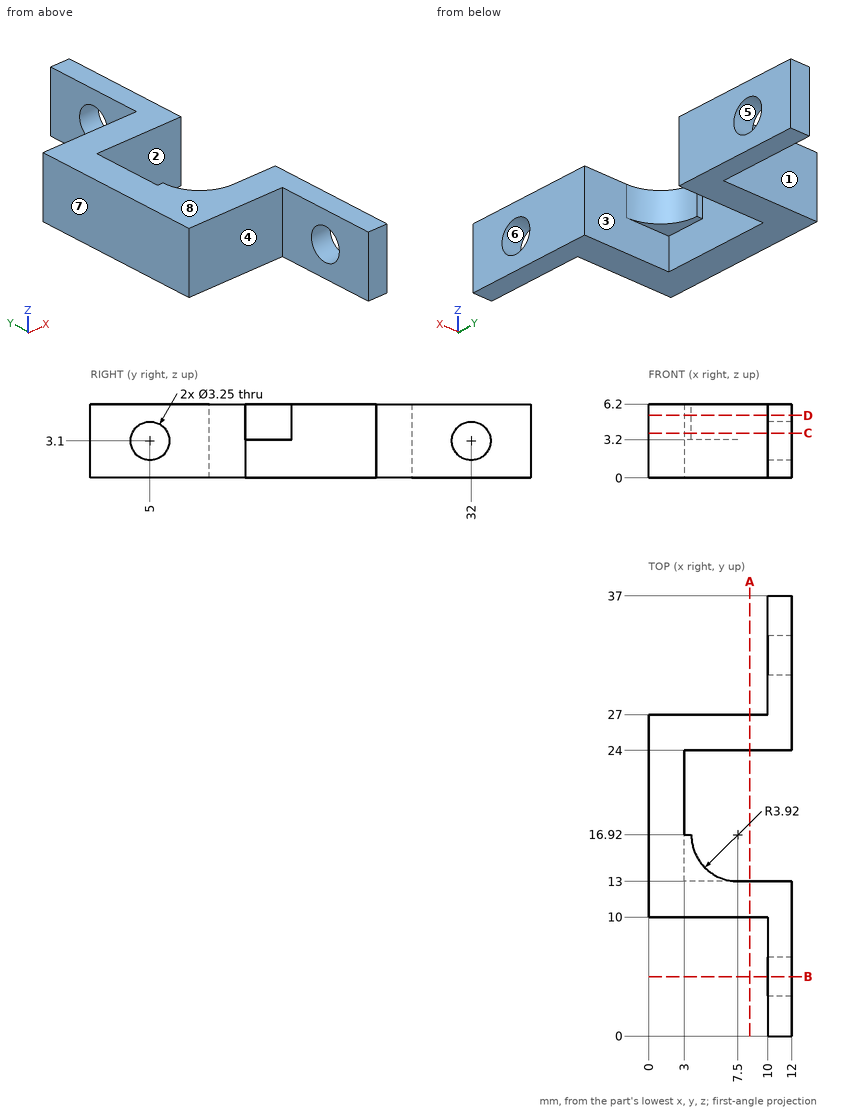
Could you check a few things on this drawing? It's one solid part, dimensions in mm from its lowest x, y, z. A direction names the side the tool comes from. Coordinates: 2 decimals unless noted, no trailing zeros. Order: outer loops, then holes, each group sorted by start corner. A loop starts at its lowest first (then second) coordinate and runs counter-clockwise, first axis right, second up. Notation, with made-up numbers: M 66,71 L 114,71 A22 cw 114,92 Z; hole C 0.25,-18.5 d10. An arc over 180 degrees is marked long. Answer as a JSON object with one key per item and string values. Group by question number.
(1) Suppose I cut it at D-D, the plane z = 5.25. Please give me the cut outline in (x, y), then the cut area to 3 significant figures.
(2) For pin 1 (2.5 mm diameter, centred on y = 5, z = 3.1, fed in from +X); pin 2 (3 mm diameter, centred on x = 6, z = 2.5, fed in from -Y); pin 3 (3 mm diameter, centred on y = 20.5, z = 2.5, fed in from +X); pin 4 (1.9 mm diameter, centred on x = 4, z = 4, fed in from +Y), each with a flat end and sliding along its axis, tell me the tip position at first contact or that it passes through.
(3) Suppose I cut it at C-C, the plane z = 3.75. Please give me the cut outline in (x, y).
(4) Suppose I cut it at A-A, the plane x = 8.5. Please give me the cut outline in (y, z), then the cut area to 3 significant figures.
(5) Suppose I cut it at B-B, the plane y = 5. Please give me the cut outline in (x, z) (3 decimals).
(6) I need wall thicknesses on probe 1 along Y at (x, z) = (9.75, 3); probe 2 along Z at (x, y) = (10.6, 5) (3 decimals); probe 3 along Y at (x, z) = (3.25, 4). Which ranges of each line are inside material? Lowest first, please.
(7) If we mould it in two halves opening along Z, with no side actions, what happens to the marked faces 6, 7 and 8? For each: released by +Z, released by -Z, zero draft, split by the parting line, or undercut.
(8) Which directions (+Z, -Z, +X, -X, +Y, -Y) give clear straight access to the entire face, cutting with the end or side of a thin tool? Please do the marked faces 1, 2, 3, 4 and 5.
Values found:
{
 "1": {"outline": "M 0,10 L 10,10 L 10,0 L 12,0 L 12,13 L 7.5,13 A3.92 cw 3.58,16.92 L 3,16.92 L 3,24 L 12,24 L 12,37 L 10,37 L 10,27 L 0,27 Z", "area": "151 mm^2"},
 "2": {"pin 1": "passes through", "pin 2": "stops at y = 10", "pin 3": "stops at x = 3", "pin 4": "stops at y = 27"},
 "3": {"outline": "M 0,10 L 10,10 L 10,6.49 L 12,6.49 L 12,13 L 7.5,13 A3.92 cw 3.58,16.92 L 3,16.92 L 3,24 L 12,24 L 12,30.51 L 10,30.51 L 10,27 L 0,27 Z; M 10,0 L 12,0 L 12,3.51 L 10,3.51 Z; M 10,33.49 L 12,33.49 L 12,37 L 10,37 Z"},
 "4": {"outline": "M 10,0 L 13,0 L 13,6.2 L 10,6.2 Z; M 24,0 L 27,0 L 27,6.2 L 24,6.2 Z", "area": "37.2 mm^2"},
 "5": {"outline": "M 10,0 L 12,0 L 12,1.475 L 10,1.475 Z; M 10,4.725 L 12,4.725 L 12,6.2 L 10,6.2 Z"},
 "6": {"probe 1": "y = 10 to 13, 24 to 27", "probe 2": "z = 0 to 1.475, 4.725 to 6.2", "probe 3": "y = 10 to 16.92, 24 to 27"},
 "7": {"face 6": "undercut", "face 7": "zero draft", "face 8": "released by +Z"},
 "8": {"face 1": "+Z, -Z, -X, +Y", "face 2": "+Z, -Z, +X", "face 3": "-Z, +X", "face 4": "+Z, -Z, -X, -Y", "face 5": "+X, -X"}
}
